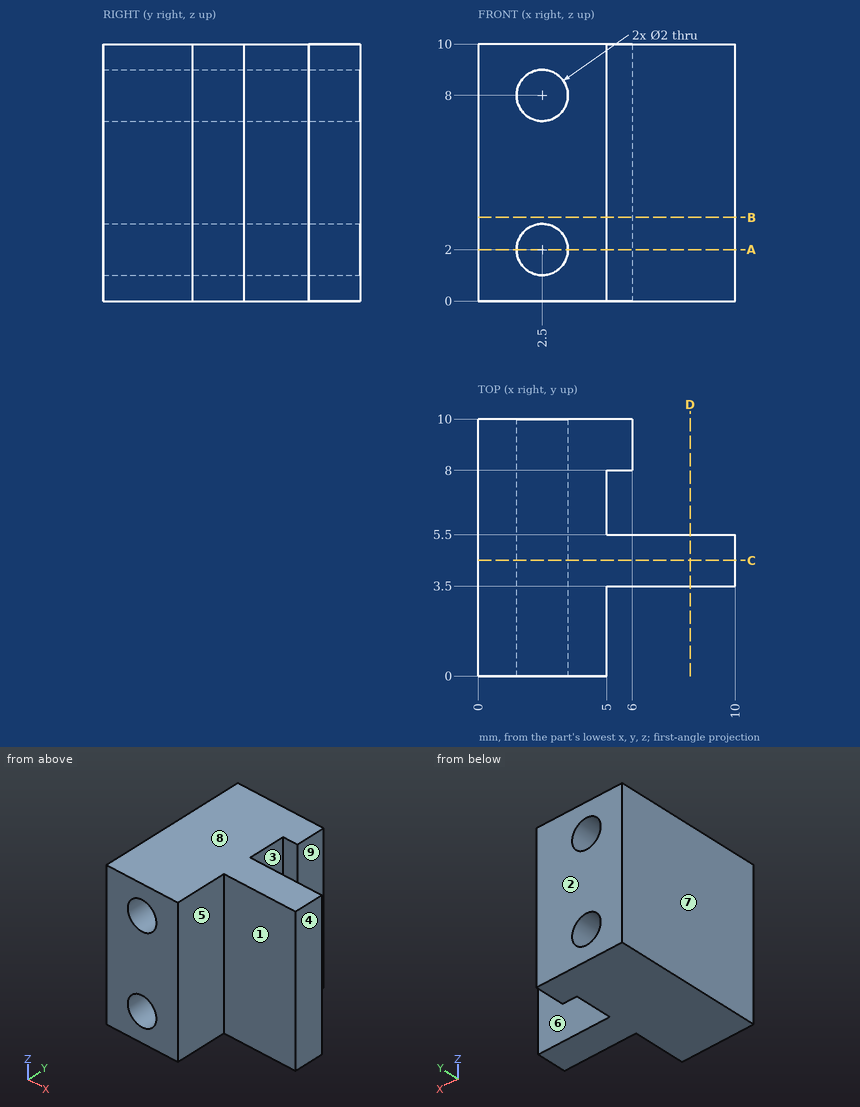
Geometry check sheet. Reference: drawing and pictorial views, mm from the part's lowest x, y, z. A direction names the side the tool comes from. Coordinates: 2 decimals unless noted, no trailing zeros. Write each loop counter-clockwise with the first axis right and the second up, starting at its lowest first coordinate (ties: lowest second). Pieces come first, ordered by that corner, then holes. Notation, with made-up numbers: (88.5, 85.5) - (123.5, 85.5) arc R23 ccw to (123.5, 96.5) - close; hole circle Ø1 at (75, 9.5). An arc over 180 degrees is marked (long way). Write item = value, one per line.
Q1. Cross-section at A-A (z = 2). Enter the section's corners in (x, y).
Answer:
outline = (0, 0) - (1.5, 0) - (1.5, 10) - (0, 10) - close; (3.5, 0) - (5, 0) - (5, 3.5) - (10, 3.5) - (10, 5.5) - (5, 5.5) - (5, 8) - (6, 8) - (6, 10) - (3.5, 10) - close
Q2. Cross-section at B-B (z = 3.25). Enter the section's corners in (x, y), plus the area to 3 significant figures.
Answer:
outline = (0, 0) - (5, 0) - (5, 3.5) - (10, 3.5) - (10, 5.5) - (5, 5.5) - (5, 8) - (6, 8) - (6, 10) - (0, 10) - close
area = 62.0 mm²
Q3. Mould release check, pull along Y, two halves, no side actions. Record for the marked faces 1, 2, 3 and 4: released by +Y, released by -Y, zero draft, split by the parting line, or undercut.
Answer:
face_1 = released by -Y
face_2 = released by +Y
face_3 = undercut
face_4 = zero draft
Q4. Material ranges on L1, parallel to Z at x = 2.5, y = 5.5; L2, parallel to Z at x = 2, y = 3.75; L3, parallel to X at y = 5, z = 8, recorded low to high. Write a range as from..to.
Answer:
L1 = 0..1, 3..7, 9..10
L2 = 0..1.13, 2.87..7.13, 8.87..10
L3 = 0..1.5, 3.5..10
Q5. Cross-section at D-D (x = 8.25). Enter the section's corners in (y, z), plus the area to 3 significant figures.
Answer:
outline = (3.5, 0) - (5.5, 0) - (5.5, 10) - (3.5, 10) - close
area = 20.0 mm²
Q6. Go/stop test with flat-tipped pins: pin 1 Ø2 at (y, z) = (8.5, 6.5) entering from +X; pin 2 Ø2.5 at (x, z) = (6.5, 5) entering from -Y; pin 3 Ø1.8 at (y, z) = (1.5, 5) entering from +X. Record where each tip stops, or that it passes through.
Answer:
pin_1 = 6
pin_2 = 3.5
pin_3 = 5
Q7. Access from +Z, -Z, +X, -X, +Y, -Y to the whole of each face (thin tool, end or side, straight path). Record for the marked faces 5, 6, 7, 8 and 9.
Answer:
face_5 = +Z, -Z, +X, -Y
face_6 = +Z, -Z, +X
face_7 = +Z, -Z, -X, +Y, -Y
face_8 = +Z, +X, -X, +Y, -Y
face_9 = +Z, -Z, +X, +Y
Q8. Cross-section at C-C (y = 4.5). Enter the section's corners in (x, z), plus the area to 3 significant figures.
Answer:
outline = (0, 0) - (10, 0) - (10, 10) - (0, 10) - close; hole circle Ø2 at (2.5, 2); hole circle Ø2 at (2.5, 8)
area = 93.7 mm²
